CAD build for the part. Positions are in the model's coordinates, mm. Face numbers are marked on the shaded views. A direction names the side the tool comes from. Coordinates: 2 decimals unless noted, no trailing zeros. Order: outer loops, then holes, each group sorted by start corner. A loop starts at its lowest first (then second) coordinate and runs counter-clockwise, first axis right, second up. Notation, with made-up numbers: (-34, -22.5) - (-22, -22.5) arc R17 cw to (-22, -6.5) - close; hole circle Ø10 at (-1, -1). An arc over 180 degrees is marked (long way). Use one line per item in the form item = value.
```python
from build123d import *

# Parameters (mm, degrees)
SKETCH_1_W      = 70
SKETCH_1_H      = 70
EXTRUDE_1_DEPTH = 70
SKETCH_4_R      = 25
EXTRUDE_2_DEPTH = 200
SKETCH_5_R      = 25
EXTRUDE_3_DEPTH = 200


with BuildPart() as part:
    # 스케치1 → 보스-돌출1 (new body)
    with BuildSketch(Plane.XY):
        Rectangle(SKETCH_1_W, SKETCH_1_H)
    extrude(amount=EXTRUDE_1_DEPTH)

    # 스케치4 → 보스-돌출2 (add)
    with BuildSketch(Plane.XY.offset(70)):
        Circle(SKETCH_4_R)
    extrude_2 = extrude(amount=EXTRUDE_2_DEPTH)

    # 대칭 복사1: 보스-돌출2 across plane
    add(extrude_2.mirror(Plane.XY.offset(35)))

    # 스케치5 → 보스-돌출3 (add)
    with BuildSketch(Plane(origin=(0, 35, 0), x_dir=(1, 0, 0), z_dir=(0, 1, 0))):
        with Locations(Location((0, -35, 0), (0, 0, 180))):
            Circle(SKETCH_5_R)
    extrude_3 = extrude(amount=EXTRUDE_3_DEPTH)

    # 대칭 복사2: 보스-돌출3 across plane
    add(extrude_3.mirror(Plane.ZX))


solid = part.part
```
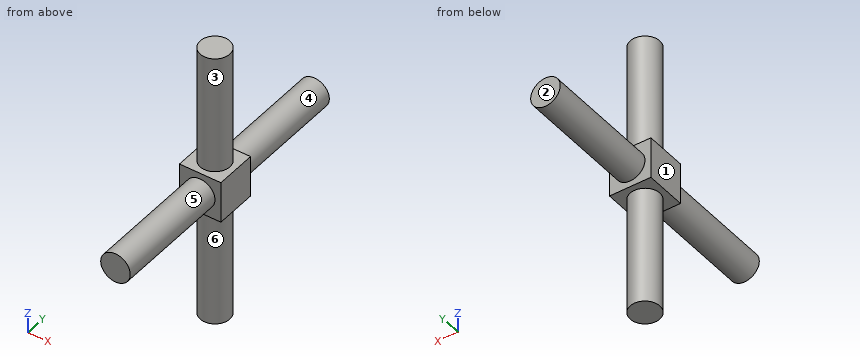
Item 1: Drop flat-ended pins along their axis: pin 1 (12 mm diameter, centred on x = -17.5, z = 99, fed in from +Y); pin 2 (1.5 mm diameter, centred on x = -15.5, z = 146.5, fed in from -Y); pin 3 (10 mm diameter, centred on x = 12, z = 218.5, fed in from +Y). Give the stop position or say it passes through.
Derived:
pin_1 = 22.2
pin_2 = -20.19
pin_3 = 24
Item 2: Two-plate mould, pull along Y, no slides. Class the marked faces 1, 2 and 3: +Y half, -Y half, draft (parallel to the pull), parting line (faces both ways), or undercut.
Derived:
face_1 = draft
face_2 = +Y half
face_3 = parting line
Item 3: Cut at A-A, the plane z = 35. Write the cut outline in (x, y), plus the area to 3 significant figures.
Derived:
outline = (-35, -35) - (-25, -35) - (-25, -235) - (25, -235) - (25, -35) - (35, -35) - (35, 35) - (25, 35) - (25, 235) - (-25, 235) - (-25, 35) - (-35, 35) - close
area = 24,900 mm²
Item 4: Cut at D-D, the plane z = 195. Write the cut outline in (x, y).
Derived:
outline = circle Ø50 at (0, 0)
Item 5: Cut at B-B, the plane y = 0. Write the cut outline in (x, z), plus the area to 3 significant figures.
Derived:
outline = (-35, 0) - (-25, 0) - (-25, -200) - (25, -200) - (25, 0) - (35, 0) - (35, 70) - (25, 70) - (25, 270) - (-25, 270) - (-25, 70) - (-35, 70) - close
area = 24,900 mm²
Item 6: Cut at C-C, the plane x = 0. Write the cut outline in (y, z).
Derived:
outline = (-235, 10) - (-35, 10) - (-35, 0) - (-25, 0) - (-25, -200) - (25, -200) - (25, 0) - (35, 0) - (35, 10) - (235, 10) - (235, 60) - (35, 60) - (35, 70) - (25, 70) - (25, 270) - (-25, 270) - (-25, 70) - (-35, 70) - (-35, 60) - (-235, 60) - close
Item 7: Drill centre lines: line 1 (Y direction, x = 21, z = 92); line 2 (Z direction, x = -22.5, y = 182); line 3 (Y direction, x = 17.5, z = 196.5). Where is each one in solid material? Low to high. Write a range as [from, to].
Derived:
line_1 = [-13.56, 13.56]
line_2 = [24.1, 45.9]
line_3 = [-17.85, 17.85]
Item 8: 3-axis set-ups, long thin cutter, end or side, ignore diameter. For the marked faces 4, 5 and 6: which of +Z, -Z, +X, -X, +Y, -Y reach the whole face in a straight line?
Derived:
face_4 = +Y
face_5 = -Y
face_6 = -Z
